Geometry check sheet. Reference: drawing and pictorial views, mm from the part's lowest x, y, z. Round coordinates to 2 decimals unless told otherwise and drop trailing zeros. Loops run counter-clockwise (first coordinate to the right, second up) from the corner with the lowest first, then second, coordinate; pieces in that order, holes last. Notation, with made-up numbers: (64, 35.25) -> (112, 35.25) arc R27 cw to (112, 59.25) -> close; hole circle Ø9 at (-5.5, 3.5). An arc over 180 degrees is marked (long way). Use one line per item in the form item = value.
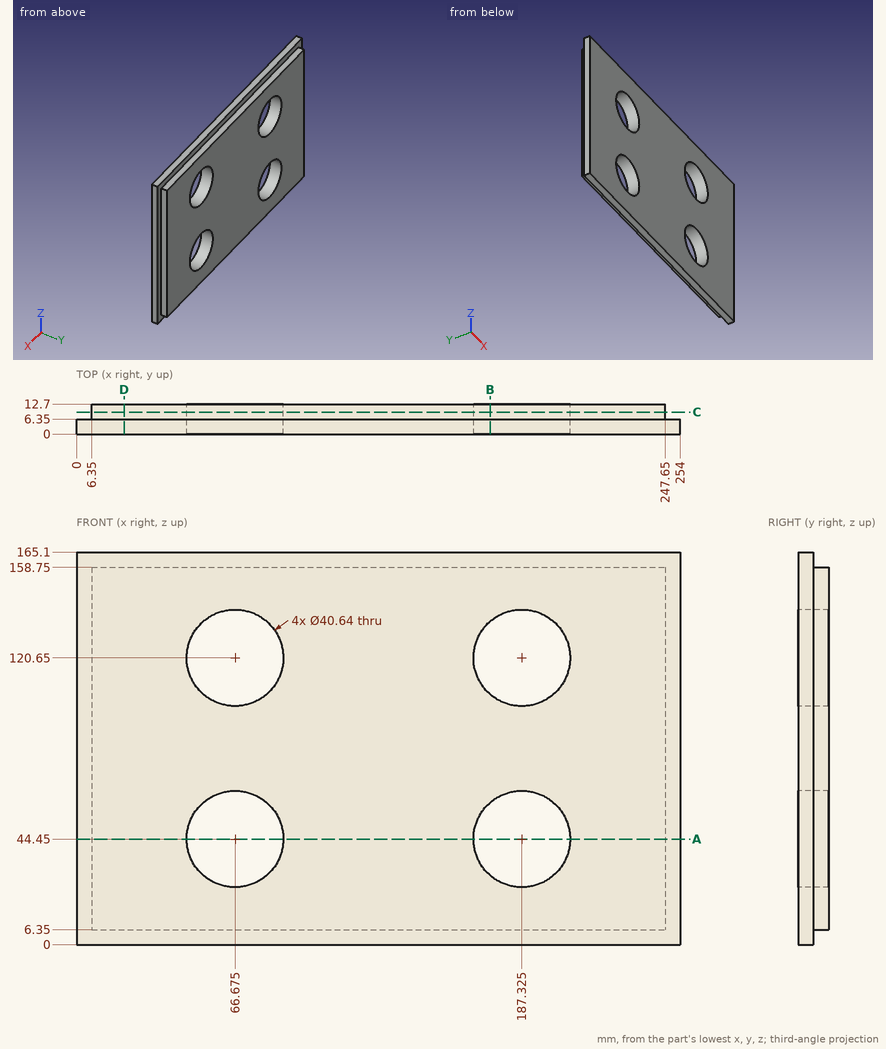
1. Material ranges on line 1 along X through (y, z) = (9.25, 45); line 2 along X through (y, z) = (4.25, 120.65) (3 decimals); line 3 along Z through (x, y) = (54, 10), recorded low to high.
Return value:
line_1 = 6.35 to 46.36, 86.99 to 167.01, 207.64 to 247.65
line_2 = 0 to 46.355, 86.995 to 167.005, 207.645 to 254
line_3 = 6.35 to 28.57, 60.33 to 104.77, 136.53 to 158.75
2. Section check C-C (y = 9.25). Record the boundary of the cut face in (x, z) (3 decimals).
Return value:
outline = (6.35, 6.35) -> (247.65, 6.35) -> (247.65, 158.75) -> (6.35, 158.75) -> close; hole circle Ø40.64 at (66.675, 44.45); hole circle Ø40.64 at (66.675, 120.65); hole circle Ø40.64 at (187.325, 44.45); hole circle Ø40.64 at (187.325, 120.65)
3. Section check A-A (z = 44.45). Record the boundary of the cut face in (x, y) (3 decimals).
Return value:
outline = (0, 0) -> (46.355, 0) -> (46.355, 12.7) -> (6.35, 12.7) -> (6.35, 6.35) -> (0, 6.35) -> close; (86.995, 0) -> (167.005, 0) -> (167.005, 12.7) -> (86.995, 12.7) -> close; (207.645, 0) -> (254, 0) -> (254, 6.35) -> (247.65, 6.35) -> (247.65, 12.7) -> (207.645, 12.7) -> close
4. Section check B-B (x = 174). Record the boundary of the cut face in (y, z).
Return value:
outline = (0, 0) -> (6.35, 0) -> (6.35, 6.35) -> (12.7, 6.35) -> (12.7, 29.11) -> (0, 29.11) -> close; (0, 59.79) -> (12.7, 59.79) -> (12.7, 105.31) -> (0, 105.31) -> close; (0, 135.99) -> (12.7, 135.99) -> (12.7, 158.75) -> (6.35, 158.75) -> (6.35, 165.1) -> (0, 165.1) -> close
5. Section check D-D (x = 20). Record the boundary of the cut face in (y, z).
Return value:
outline = (0, 0) -> (6.35, 0) -> (6.35, 6.35) -> (12.7, 6.35) -> (12.7, 158.75) -> (6.35, 158.75) -> (6.35, 165.1) -> (0, 165.1) -> close
6. Gauge pin test, flat ends, axial feed: pin 1 (7 mm diameter, centred on x = 101, y = 10.5, fed in from -Z); pin 2 (1 mm diameter, centred on y = 11, z = 82.5, fed in from +X); pin 3 (24.5 mm diameter, centred on x = 66.675, z = 120.65, fed in from +Y). Record the tip position at first contact, or that the pin passes through.
Return value:
pin_1 = 6.35
pin_2 = 247.65
pin_3 = through
